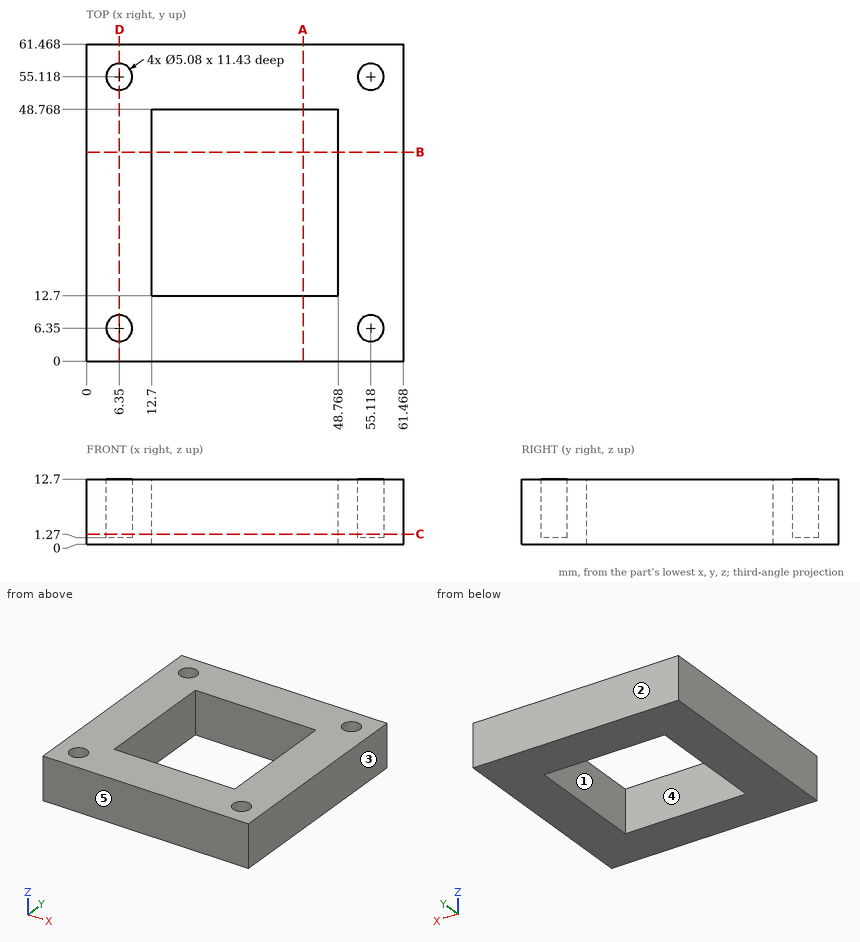
The figure shows three views and two pictorial views of one solid part (mm, origin at its lowest corner). Answer the questions. A direction names the side the tool comes from. Round coordinates to 2 decimals unless told otherwise and drop trailing zeros. Write each loop counter-clockwise with the first axis right and the second up, starting at its lowest first coordinate (ties: lowest second). Pieces come first, ordered by that corner, then holes. Notation, with made-up numbers: M 19,3 L 52,3 A32 ccw 52,31 Z; hole C 78.5,-38.75 d1. An arc over 180 degrees is marked long. Write each question's results on one line, items separated by ' | '. Start each with the question number.
(1) This flat-tipped pin is pushed along its axis until it touches: P1, Ø2.5, axis at x = 6, y = 7, coming from the +Z side. Where does it stop, or does it pass through?
(2) Find the intervals of material crossed by line 1 (Y direction, x = 6.35, z = 8.75); line 2 (X direction, y = 34.5, z = 0.75), in increasing order.
(3) The part is cut by section A-A, the plane x = 42. Write down the section's boundary in (y, z).
(4) The part is cut by section C-C, the plane z = 2. Write down the section's boundary in (x, y), and give its area (3 significant figures).
(5) For the marked faces 4 and 5, determine the directions among +Z, -Z, +X, -X, +Y, -Y from which every point of the face is accessible in a straight line to the end or side of a thin tool.
(6) Determine the mould class of the marked faces 1, 2 and 3 for opening direction Y: +Y half, -Y half, draft (parallel to the pull), parting line (faces both ways), or undercut.
(7) The part is cut by section D-D, the plane x = 6.35. Write down the section's boundary in (y, z), and give its area (3 significant figures).
Worked answers:
1) P1: stops at z = 1.27
2) line 1: y = 0 to 3.81, 8.89 to 52.58, 57.66 to 61.47 | line 2: x = 0 to 12.7, 48.77 to 61.47
3) outline: M 0,0 L 12.7,0 L 12.7,12.7 L 0,12.7 Z; M 48.77,0 L 61.47,0 L 61.47,12.7 L 48.77,12.7 Z
4) outline: M 0,0 L 61.47,0 L 61.47,61.47 L 0,61.47 Z; hole C 6.35,6.35 d5.08; hole C 6.35,55.12 d5.08; hole M 12.7,12.7 L 48.77,12.7 L 48.77,48.77 L 12.7,48.77 Z; hole C 55.12,6.35 d5.08; hole C 55.12,55.12 d5.08 | area: 2,400 mm²
5) face 4: +Z, -Z | face 5: +Z, -Z, +X, -X, -Y
6) face 1: undercut | face 2: +Y half | face 3: draft
7) outline: M 0,0 L 61.47,0 L 61.47,12.7 L 57.66,12.7 L 57.66,1.27 L 52.58,1.27 L 52.58,12.7 L 8.89,12.7 L 8.89,1.27 L 3.81,1.27 L 3.81,12.7 L 0,12.7 Z | area: 665 mm²
